Check sheet for the modelled part. Datum: model origin and axes. Units: mm. A direction names the side the tool comes from. Round coordinates to 2 decimals unless told otherwise and drop trailing zeros. Loops run counter-clockwise (first coordinate to the right, second up) from the corner with the lowest first, then second, coordinate; pieces in that order, holes last. Notation, with made-up numbers: (60.5, 81.5) -> (78.5, 81.5) arc R27 cw to (78.5, 118.5) -> close; hole circle Ø8 at (26.25, 21). An arc over 180 degrees is marked (long way). One line per item, written item: value. Start each with the question number.
1. Set-up check for faces 5 (the face through (17, -25, 20)), 6 (the face through (17, -11, 7.162)), 7 (the face through (25.53, -22.54, 18.36)): record each of +Z, -Z, +X, -X, +Y, -Y from which the full face is reachable in a straight line by a thin tool's end or side.
2. Release check for a two-part mould opening along X. For faces 1 (the face through (17, 0, 16)), 2 (the face through (24, -20, 22)), 3 (the face through (16.072, -22.535, 19.156)), 4 (the face through (34.653, -12, 16)) record: +X half, -X half, draft (parallel to the pull), parting line (faces both ways), or undercut.
3. Cross-section at C-C on x = 27. Record the cut outline in (y, z), then the cut area to 3 significant figures.
4. Material ranges on L1, parallel to X at y = -11, z = 12.5; L2, parallel to Z at x = 13, y = -10.5; L3, parallel to Y at x = 24.5, z = 26, recorded low to high.
5. Cross-section at B-B on y = -22.75. Record the cut outline in (x, z), then the cut area to 3 significant figures.
6. Cross-section at A-A on z = 25. Record the cut outline in (x, y).
7. Cross-section at D-D on z = 19.5. Record the cut outline in (x, y).
8. Go/stop test with flat-tipped pins: pin 1 (8 mm diameter, centred on x = 19, y = -9.5, fed in from +Z); pin 2 (4.5 mm diameter, centred on x = 13.38, z = 14.94, fed in from -Y); pin 3 (8 mm diameter, centred on x = 26.62, z = 23.24, fed in from -Y). Record where each tip stops, or that it passes through.
from build123d import *

# Parameters (mm, degrees)
F0_W           = 34.65341
F0_H           = 32.161761
F1_DEPTH       = 25
F2_R           = 6.731934
F3_DEPTH       = 25
F5_D           = 5
F5_CBORE_D     = 10
F5_CBORE_DEPTH = 5


with BuildPart() as f1:
    # F0 (on Front) → F1 (new body)
    with BuildSketch(Plane.XZ):
        with Locations((17.326705, 16.08088)):
            Rectangle(F0_W, F0_H)
    extrude(amount=F1_DEPTH)

    # F2 (on face) → F3 (cut)
    with BuildSketch(Plane.XY.offset(32.161761)):
        with Locations((17.258551, -11.357421)):
            Circle(F2_R)
    extrude(amount=-F3_DEPTH, mode=Mode.SUBTRACT)

    # F5 (through all)
    with Locations(Plane.XZ.offset(25)):
        with Locations((13.383781, 14.940267), (26.61572, 23.240186), (22.894813, 8.254618)):
            CounterBoreHole(F5_D / 2, F5_CBORE_D / 2, F5_CBORE_DEPTH)


solid = f1.part
Taken from the geometry:
1. face 5: +Z, -Z, +X, -X, -Y
1. face 6: +Z
1. face 7: -Y
2. face 1: draft
2. face 2: undercut
2. face 3: undercut
2. face 4: +X half
3. outline: (-25, 0) -> (0, 0) -> (0, 20.77) -> (-20, 20.77) -> (-20, 18.25) -> (-25, 18.25) -> (-25, 11.11) -> (-20, 11.11) -> (-20, 5.4) -> (-25, 5.4) -> close; (-25, 28.23) -> (-20, 28.23) -> (-20, 25.71) -> (0, 25.71) -> (0, 32.16) -> (-25, 32.16) -> close
3. area: 627 mm2
4. L1: x = 0 to 10.54, 23.98 to 34.65
4. L2: z = 0 to 7.16
4. L3: y = -20 to 0
5. outline: (0, 0) -> (34.65, 0) -> (34.65, 32.16) -> (0, 32.16) -> close; hole circle Ø10 at (13.38, 14.94); hole circle Ø10 at (22.89, 8.25); hole circle Ø10 at (26.62, 23.24)
5. area: 879 mm2
6. outline: (0, -25) -> (21.94, -25) -> (21.94, -20) -> (24.84, -20) -> (24.84, 0) -> (0, 0) -> close; (28.39, -20) -> (31.3, -20) -> (31.3, -25) -> (34.65, -25) -> (34.65, 0) -> (28.39, 0) -> close; hole circle Ø13.46 at (17.26, -11.36)
7. outline: (0, -25) -> (11.33, -25) -> (11.33, -20) -> (15.44, -20) -> (15.44, -25) -> (23.3, -25) -> (23.3, -20) -> (29.93, -20) -> (29.93, -25) -> (34.65, -25) -> (34.65, 0) -> (0, 0) -> close; hole circle Ø13.46 at (17.26, -11.36)
8. pin 1: stops at z = 7.16
8. pin 2: passes through
8. pin 3: stops at y = -20
